Autodesk Inventor part; units mm, degrees
ref_plane "YZ Plane" through (0, 0, 0) normal (1, 0, 0) x (0, 1, 0)
ref_plane "XZ Plane" through (0, 0, 0) normal (0, 1, 0) x (-1, 0, 0)
ref_plane "XY Plane" through (0, 0, 0) normal (0, 0, 1) x (1, 0, 0)
sketch "스케치1" plane through (0, 0, 0) normal (0, 1, 0) x (-1, 0, 0)
  line L0 (0, 0) -> (11.4, 0)
  line L1 (11.4, 0) -> (11.4, -27.5)
  line L2 (11.4, -27.5) -> (0, -27.5)
  line L3 (0, -27.5) -> (0, 0)
  dimension "d0" = 11.4
  dimension "d1" = 27.5
extrude "돌출1" add sketch "스케치1" along normal blind 1.5
fillet "모깎기1" radius 2 2 edges at (-11.4, 0, -13.75) (0, 0, -13.75)
sketch "스케치4" plane through (0, 1.5, 0) normal (0, 1, 0) x (1, 0, 0)
  line L0 (-11.4, 27.5) -> (-11.4, 0)
  line L1 (0, 0) -> (0, 27.5)
  line L2 (0, 27.5) -> (-11.4, 27.5)
  line L3 (-11.4, 27.5) -> (0, 27.5)
  line L4 (0, 27.5) -> (0, 26.5)
  line L5 (0, 26.5) -> (-11.4, 26.5)
  line L6 (-11.4, 26.5) -> (-11.4, 27.5)
  line L7 (-1.2, 26.5) -> (-1.2, 27.5)
  dimension "d18" = 1
  dimension "d21" = 1.2
extrude "돌출4" add sketch "스케치4" along normal blind 1.2 contours L2 L7 L5 L0
properties part number "_3D 인쇄"
For this review, take the finished solid that the model builds, in its own axes (mm). A direction names the side the tool comes from. Give positions to 0.01 mm unless a question says otherwise; leave off trailing zeros. Write each loop counter-clockwise with the first axis right and the second up, starting at its lowest first coordinate (ties: lowest second). Pieces come first, ordered by that corner, then holes. Notation, with made-up numbers: (45, 27) -> (99, 27) arc R12 cw to (99, 41) -> close; hole circle Ø5 at (-29, -32.5). An arc over 180 degrees is marked (long way). Use CSV: the item, a comma, the result in double quotes.
Q1. Tool access review of faces 1 (the face through (-6, 2.7, -27)), 2 (the face through (-6, 2, -26.5)), 3 (the face through (-1.2, 2, -27)): name each direction out of +Z, -Z, +X, -X, +Y, -Y from which nothing blocks a thin tool from reaching the whole face with its end or side.
Conclusion:
face 1,"+Z, -Z, +X, -X, +Y"
face 2,"+Z, +X, -X, +Y"
face 3,"+Z, -Z, +X, +Y"
Q2. Take a section at B-B, the plane x = -6.75. Write out the cut boundary in (y, z).
Conclusion:
outline,"(0, -27.5) -> (2.7, -27.5) -> (2.7, -26.5) -> (1.5, -26.5) -> (1.5, 0) -> (0, 0) -> close"
Q3. For P1, Ø4, axis at x = -8, z = -11, coming from the +Y side; P2, Ø1, axis at x = -4, y = 2.5, coming from the +Z side, all flat-tipped, find the tip position at first contact; note any pin that passes through.
Conclusion:
P1,"y = 1.5"
P2,"z = -26.5"
Q4. Take a section at A-A, the plane z = -15. Write out the cut boundary in (x, y).
Conclusion:
outline,"(-11.4, 1.5) arc R2 ccw to (-9.46, 0) -> (-1.94, 0) arc R2 ccw to (0, 1.5) -> close"
Q5. Take a section at D-D, the plane x = -1.5. Write out the cut boundary in (y, z).
Conclusion:
outline,"(0.05, -27.5) -> (2.7, -27.5) -> (2.7, -26.5) -> (1.5, -26.5) -> (1.5, 0) -> (0.05, 0) -> close"
Q6. Take a section at C-C, the plane y = 2.3. Write out the cut boundary in (x, z), then the cut area to 3 significant figures.
Conclusion:
outline,"(-11.4, -27.5) -> (-1.2, -27.5) -> (-1.2, -26.5) -> (-11.4, -26.5) -> close"
area,"10.2 mm2"
Q7. To check wall thickness, follow probe 1 along Y at (x, z) = (-3, -21.5); probe 2 along Z at (x, y) = (-10, 1.95); probe 3 along X at (y, z) = (1.2, -4.75). State the ranges of each line that lie inside material, in increasing order. Write a range as [from, to].
Conclusion:
probe 1,"[0, 1.5]"
probe 2,"[-27.5, -26.5]"
probe 3,"[-11.3, -0.1]"
